Autodesk Inventor part; units mm, degrees
ref_plane "YZ Plane" through (0, 0, 0) normal (1, 0, 0) x (0, 1, 0)
ref_plane "XZ Plane" through (0, 0, 0) normal (0, 1, 0) x (-1, 0, 0)
ref_plane "XY Plane" through (0, 0, 0) normal (0, 0, 1) x (1, 0, 0)
sketch "Sketch1" plane through (0, 0, 0) normal (1, 0, 0) x (0, 1, 0)
  line L0 (20, 57) -> (-20, 57)
  line L1 (-20, 57) -> (-20, -57)
  line L2 (-20, -57) -> (20, -57)
  line L3 (20, -57) -> (20, 57)
  line L4 (20, 57) -> (-20, -57) construction
  line L5 (-20, 57) -> (20, -57) construction
  line L6 (-17, 54) -> (17, 54)
  line L7 (17, 54) -> (17, -54)
  line L8 (17, -54) -> (-17, -54)
  line L9 (-17, -54) -> (-17, 54)
  line L10 (-17, 54) -> (17, -54) construction
  line L11 (17, 54) -> (-17, -54) construction
  point P0 (0, 0)
  point P1 (0, -57)
  point P2 (0, -54)
  dimension "d0" = 114
  dimension "d1" = 40
  dimension "d2" = 3
  dimension "d3" = 3
extrude "Extrusion1" add sketch "Sketch1" along normal blind 300
sketch "Sketch2" plane through (0, 20, 57) normal (0, 1, 0) x (1, 0, 0)
  line L0 (300, 114) -> (300, 0)
  circle A0 centre (300, 57) radius 54
  point P0 (0, 57)
  point P1 (300, 111)
  point P2 (300, 3)
extrude "Extrusion2" cut sketch "Sketch2" against normal through all contours L0 A0 picked at (282.6871, 52.0741)
sketch "Sketch3" plane through (0, -20, 57) normal (0, 0, 1) x (1, 0, 0)
  circle A0 centre (20, 20) radius 4
  line L0 (0, 40) -> (0, 0)
  point P0 (0, 20)
  point P1 (0, 20)
  dimension "d8" = 8
  dimension "d9" = 20
extrude "Extrusion3" cut sketch "Sketch3" against normal through all
properties part number "AirIntake"
Work out the finished part from the listing and answer in its coordinate system (mm). A direction names the side the tool comes from. Give positions to 0.01 mm unless a question says otherwise; leave off trailing zeros. Loops run counter-clockwise (first coordinate to the right, second up) from the corner with the lowest first, then second, coordinate; pieces in that order, holes last. Notation, with made-up numbers: (-26.75, 27.5) - (17.25, 27.5) arc R16 ccw to (17.25, 33.5) - close; hole circle Ø8 at (57, 12). An arc over 180 degrees is marked (long way). Answer in a Markdown table with one row per item. Add a question column.
Q1. Determine the mould class of faces 1 (the flat face through (0, -18, 4)), 2 (the flat face through (115, -17, -1)), 3 (the flat face through (115, 20, -1)) for opening direction Y: released by +Y, released by -Y, zero draft, split by the parting line, or undercut.
Q2. The part is cut by section D-D (y = 0). Determine the outline of the cut face in (x, z).
Q3. The part is cut by section C-C (x = 185.5). Determine the outline of the cut face in (y, z).
Q4. A tool of negligible diameter and unlimited length cuts with its end or side. For faces 4 (the flat face through (148, 0, 54)), 5 (the flat face through (148, 0, -57)), from which of +Z, -Z, +X, -X, +Y, -Y can it reach the whole face along a straight path? Write none if from no direction.
Q5. This flat-tipped pin is pushed along its axis until it touches: P1, Ø6.5, axis at x = 20, y = 0, coming from the +Z side. Where does it stop, or does it pass through?
Q6. Consider line 1 along Y through (x, z) = (20, -55.65); line 2 along Z through (x, y) = (144.5, 13.5); line 3 along Y through (x, z) = (39, -30.5). Determine where each line is inside the solid, lowest interval first.
Q7. The part is cut by section A-A (x = 20). Determine the outline of the cut face in (y, z).
Q8. The part is cut by section B-B (z = 0). Determine the outline of the cut face in (x, y), and give its area (3 significant figures).
Solution:
| question | item | result |
|---|---|---|
| 1 | face 1 | zero draft |
| 1 | face 2 | undercut |
| 1 | face 3 | released by +Y |
| 2 | outline | (0, -57) - (16, -57) - (16, -54) - (0, -54) - close; (0, 54) - (16, 54) - (16, 57) - (0, 57) - close; (24, -57) - (300, -57) - (300, -54) - (24, -54) - close; (24, 54) - (300, 54) - (300, 57) - (24, 57) - close |
| 3 | outline | (-20, -57) - (20, -57) - (20, 57) - (-20, 57) - close; hole (-17, -54) - (17, -54) - (17, 54) - (-17, 54) - close |
| 4 | face 4 | +X, -X |
| 4 | face 5 | -Z, +X, -X, +Y, -Y |
| 5 | P1 | passes through |
| 6 | line 1 | y = -20 to -4, 4 to 20 |
| 6 | line 2 | z = -57 to -54, 54 to 57 |
| 6 | line 3 | y = -20 to -17, 17 to 20 |
| 7 | outline | (-20, -57) - (-4, -57) - (-4, -54) - (-17, -54) - (-17, 54) - (-4, 54) - (-4, 57) - (-20, 57) - close; (4, -57) - (20, -57) - (20, 57) - (4, 57) - (4, 54) - (17, 54) - (17, -54) - (4, -54) - close |
| 8 | outline | (0, -20) - (246, -20) - (246, -17) - (0, -17) - close; (0, 17) - (246, 17) - (246, 20) - (0, 20) - close |
| 8 | area | 1,480 mm² |
